Could you check a few things on this model? Use its own coordinates, in mm. Coordinates: 2 decimals unless noted, no trailing zeros. Loops run counter-clockwise (first coordinate to the right, second up) from the corner with the lowest first, then second, coordinate; pieces in that order, holes last.
1) Imagine slicing it at B-B on z = 40. Please give me the cut outline in (x, y), plus the area to 4 significant figures.
2) If I drill on line 1 along X through (y, z) = (1.2, 40); line 2 along Z through (x, y) = (37.5, 0.75); line 3 along X through (y, z) = (1.25, 45.5), over which ranges is the centre line in solid material (lowest first)?
3) Imagine slicing it at A-A on x = -37.5. Please give me the cut outline in (y, z).
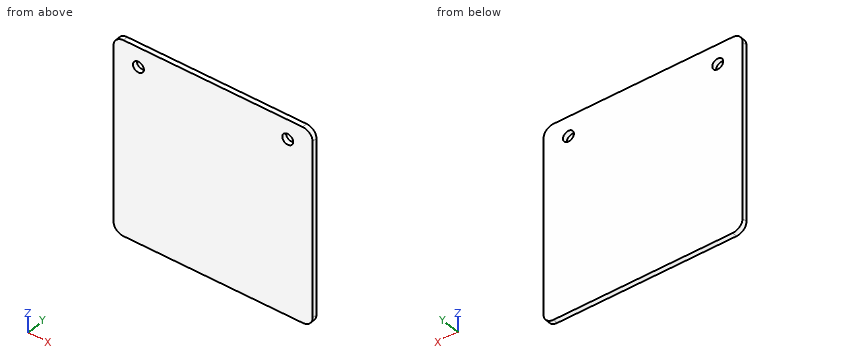
```python
from build123d import *

# Parameters (mm, degrees)
SKETCH1_W                = 100
SKETCH1_H                = 100
BOSS_EXTRUDE1_DEPTH      = 2.5
M5_CLEARANCE_HOLE1_D     = 5.5
M5_CLEARANCE_HOLE1_DEPTH = 12
M5_CLEARANCE_HOLE1_TIP   = 1.652366702
FILLET1_R                = 5


with BuildPart() as part:
    # Sketch1 → Boss-Extrude1 (new body)
    with BuildSketch(Plane(origin=(0, 0, 0), x_dir=(1, 0, 0), z_dir=(0, 1, 0))):
        Rectangle(SKETCH1_W, SKETCH1_H)
    extrude(amount=BOSS_EXTRUDE1_DEPTH)

    # M5 Clearance Hole1
    with Locations(Plane(origin=(0, 2.5, 0), x_dir=(1, 0, 0), z_dir=(0, 1, 0))):
        with Locations((-37.5, -40), (37.5, -40)):
            Hole(M5_CLEARANCE_HOLE1_D / 2, depth=M5_CLEARANCE_HOLE1_DEPTH)
            with Locations((0, 0, -(M5_CLEARANCE_HOLE1_DEPTH + M5_CLEARANCE_HOLE1_TIP / 2))):  # 118° drill point
                Cone(0, M5_CLEARANCE_HOLE1_D / 2, M5_CLEARANCE_HOLE1_TIP, mode=Mode.SUBTRACT)

    # Fillet1
    fillet1_edges = [part.edges().sort_by_distance(p)[0] for p in [
        (50, 1.25, 50),
        (-50, 1.25, 50),
        (-50, 1.25, -50),
        (50, 1.25, -50),
    ]]
    fillet(fillet1_edges, radius=FILLET1_R)


solid = part.part
```
Filled in:
1. outline: (-50, 0) - (-40.25, 0) - (-40.25, 2.5) - (-50, 2.5) - close; (-34.75, 0) - (34.75, 0) - (34.75, 2.5) - (-34.75, 2.5) - close; (40.25, 0) - (50, 0) - (50, 2.5) - (40.25, 2.5) - close
1. area: 222.5 mm2
2. line 1: x = -50 to -40.25, -34.75 to 34.75, 40.25 to 50
2. line 2: z = -50 to 37.25, 42.75 to 50
2. line 3: x = -49.97 to 49.97
3. outline: (0, -50) - (2.5, -50) - (2.5, 37.25) - (0, 37.25) - close; (0, 42.75) - (2.5, 42.75) - (2.5, 50) - (0, 50) - close
